Source: CAD feature listing. Evaluate the final solid. Frame: model axes, mm. A direction names the side the tool comes from. Round coordinates to 2 decimals unless told otherwise and drop trailing zeros. Loops run counter-clockwise (first coordinate to the right, second up) from the corner with the lowest first, then second, coordinate; pieces in that order, holes last. Notation, with made-up numbers: (-6.75, 1.25) - (3.25, 1.25) arc R27 ccw to (3.25, 37.25) - close; hole circle Ø11 at (-14.5, -28.5). An arc over 180 degrees is marked (long way). One line per question, with ' | ' between items.
from build123d import *

# Parameters (mm, degrees)
EXTRUDE_1_DEPTH     = 20
CUT_EXTRUDE_1_REACH = 71.771
SKETCH_2_R          = 1.55
SKETCH_2_R_2        = 11.5
CUT_EXTRUDE_2_REACH = 71.771
SKETCH_3_R          = 1.55
FILLET_1_R          = 5


with BuildPart() as part:
    # 草图1 → 凸台-拉伸1 (new, symmetric)
    with BuildSketch(Plane(origin=(0, 0, 0), x_dir=(0, 0, -1), z_dir=(1, 0, 0))):
        Polygon((0, 0), (0, 52), (3, 52), (3, 3), (42, 3), (42, 0), align=None)
    extrude(amount=EXTRUDE_1_DEPTH, both=True)

    # 草图2 → 切除-拉伸1 (cut, up to next)
    with BuildSketch(Plane.XY, mode=Mode.PRIVATE) as cut_extrude_1_sk1:
        with Locations((15.5, 46.5)):
            Circle(SKETCH_2_R)
    cut_extrude_1_tool1 = extrude(cut_extrude_1_sk1.sketch, amount=-CUT_EXTRUDE_1_REACH, mode=Mode.PRIVATE) & part.part
    # 草图2 → 切除-拉伸1 (cut, up to next)
    with BuildSketch(Plane.XY, mode=Mode.PRIVATE) as cut_extrude_1_sk2:
        with Locations((15.5, 15.5)):
            Circle(SKETCH_2_R)
    cut_extrude_1_tool2 = extrude(cut_extrude_1_sk2.sketch, amount=-CUT_EXTRUDE_1_REACH, mode=Mode.PRIVATE) & part.part
    # 草图2 → 切除-拉伸1 (cut, up to next)
    with BuildSketch(Plane.XY, mode=Mode.PRIVATE) as cut_extrude_1_sk3:
        with Locations(Location((-15.5, 15.5, 0), (0, 0, 90))):
            Circle(SKETCH_2_R)
    cut_extrude_1_tool3 = extrude(cut_extrude_1_sk3.sketch, amount=-CUT_EXTRUDE_1_REACH, mode=Mode.PRIVATE) & part.part
    # 草图2 → 切除-拉伸1 (cut, up to next)
    with BuildSketch(Plane.XY, mode=Mode.PRIVATE) as cut_extrude_1_sk4:
        with Locations(Location((-15.5, 46.5, 0), (0, 0, 90))):
            Circle(SKETCH_2_R)
    cut_extrude_1_tool4 = extrude(cut_extrude_1_sk4.sketch, amount=-CUT_EXTRUDE_1_REACH, mode=Mode.PRIVATE) & part.part
    # 草图2 → 切除-拉伸1 (cut, up to next)
    with BuildSketch(Plane.XY, mode=Mode.PRIVATE) as cut_extrude_1_sk5:
        with Locations((0, 31)):
            Circle(SKETCH_2_R_2)
    cut_extrude_1_tool5 = extrude(cut_extrude_1_sk5.sketch, amount=-CUT_EXTRUDE_1_REACH, mode=Mode.PRIVATE) & part.part
    add(cut_extrude_1_tool1.solids().sort_by_distance((15.5, 46.5, 0))[0], mode=Mode.SUBTRACT)
    add(cut_extrude_1_tool2.solids().sort_by_distance((15.5, 15.5, 0))[0], mode=Mode.SUBTRACT)
    add(cut_extrude_1_tool3.solids().sort_by_distance((-15.5, 15.5, 0))[0], mode=Mode.SUBTRACT)
    add(cut_extrude_1_tool4.solids().sort_by_distance((-15.5, 46.5, 0))[0], mode=Mode.SUBTRACT)
    add(cut_extrude_1_tool5.solids().sort_by_distance((0, 31, 0))[0], mode=Mode.SUBTRACT)

    # 草图3 → 切除-拉伸2 (cut, up to next)
    with BuildSketch(Plane(origin=(0, 0, 0), x_dir=(1, 0, 0), z_dir=(0, 1, 0)), mode=Mode.PRIVATE) as cut_extrude_2_sk1:
        with Locations(Location((15, 33, 0), (0, 0, 270))):
            Circle(SKETCH_3_R)
    cut_extrude_2_tool1 = extrude(cut_extrude_2_sk1.sketch, amount=CUT_EXTRUDE_2_REACH, mode=Mode.PRIVATE) & part.part
    # 草图3 → 切除-拉伸2 (cut, up to next)
    with BuildSketch(Plane(origin=(0, 0, 0), x_dir=(1, 0, 0), z_dir=(0, 1, 0)), mode=Mode.PRIVATE) as cut_extrude_2_sk2:
        with Locations(Location((15, 9, 0), (0, 0, 270))):
            Circle(SKETCH_3_R)
    cut_extrude_2_tool2 = extrude(cut_extrude_2_sk2.sketch, amount=CUT_EXTRUDE_2_REACH, mode=Mode.PRIVATE) & part.part
    # 草图3 → 切除-拉伸2 (cut, up to next)
    with BuildSketch(Plane(origin=(0, 0, 0), x_dir=(1, 0, 0), z_dir=(0, 1, 0)), mode=Mode.PRIVATE) as cut_extrude_2_sk3:
        with Locations(Location((-15, 9, 0), (0, 0, 90))):
            Circle(SKETCH_3_R)
    cut_extrude_2_tool3 = extrude(cut_extrude_2_sk3.sketch, amount=CUT_EXTRUDE_2_REACH, mode=Mode.PRIVATE) & part.part
    # 草图3 → 切除-拉伸2 (cut, up to next)
    with BuildSketch(Plane(origin=(0, 0, 0), x_dir=(1, 0, 0), z_dir=(0, 1, 0)), mode=Mode.PRIVATE) as cut_extrude_2_sk4:
        with Locations(Location((-15, 33, 0), (0, 0, 90))):
            Circle(SKETCH_3_R)
    cut_extrude_2_tool4 = extrude(cut_extrude_2_sk4.sketch, amount=CUT_EXTRUDE_2_REACH, mode=Mode.PRIVATE) & part.part
    add(cut_extrude_2_tool1.solids().sort_by_distance((15, 0, -33))[0], mode=Mode.SUBTRACT)
    add(cut_extrude_2_tool2.solids().sort_by_distance((15, 0, -9))[0], mode=Mode.SUBTRACT)
    add(cut_extrude_2_tool3.solids().sort_by_distance((-15, 0, -9))[0], mode=Mode.SUBTRACT)
    add(cut_extrude_2_tool4.solids().sort_by_distance((-15, 0, -33))[0], mode=Mode.SUBTRACT)

    # 圆角1
    fillet_1_edges = [part.edges().sort_by_distance(p)[0] for p in [
        (-20, 52, -1.5),
        (20, 52, -1.5),
        (20, 1.5, -42),
        (-20, 1.5, -42),
    ]]
    fillet(fillet_1_edges, radius=FILLET_1_R)


solid = part.part
1. Contact query for flat-ended pins moving along their axis: P1, Ø1, axis at x = 4, z = -30, coming from the -Y side; P2, Ø19.5, axis at x = -3, z = -27.5, coming from the +Y side; P3, Ø1, axis at x = 13, y = 18, coming from the -Z side. Output: stop coordinate, or through.
Worked out:
P1: stops at y = 0 | P2: stops at y = 3 | P3: stops at z = -3
2. Access query for faces 5 (the flat face through (-9, 22, -3)), 6 (the flat face through (-4, 20, 0)). Directions: +Z, -Z, +X, -X, +Y, -Y. A direction counts if a zero-diameter tool reaches every point of the face in a straight line with its end or side. Return the directions, or none.
Worked out:
face 5: -Z, +X, -X, +Y | face 6: +Z, +X, -X, +Y, -Y
3. Mould query, pull axis Y, two halves, no side actions, for faces 1 (the flat face through (0, 3, -22)), 2 (the cylindrical face through (-15.466, 1.479, -34.478)), 3 (the cylindrical face through (14.36, 16.55, -1.48)), 4 (the cylindrical face through (15.164, 44.987, -1.479)). Classes: released by +Y, released by -Y, zero draft, split by the parting line, or undercut.
Worked out:
face 1: released by +Y | face 2: zero draft | face 3: undercut | face 4: undercut
4. Section query A-A, the plane x = 0. Return loops of the section in (y, z), plus the area to 3 significant figures.
Worked out:
outline: (0, -42) - (3, -42) - (3, -3) - (19.5, -3) - (19.5, 0) - (0, 0) - close; (42.5, -3) - (52, -3) - (52, 0) - (42.5, 0) - close | area: 204 mm2
5. Material intervals for probe 1 along X at (y, z) = (0.7, -9); probe 2 along Z at (x, y) = (-15, 1); probe 3 along Y at (x, z) = (-15, -1), sorted ascending.
Worked out:
probe 1: x = -20 to -16.55, -13.45 to 13.45, 16.55 to 20 | probe 2: z = -42 to -34.55, -31.45 to -10.55, -7.45 to 0 | probe 3: y = 0 to 14.03, 16.97 to 45.03, 47.97 to 52
6. Section query D-D, the plane x = -4. Return loops of the section in (y, z), plus the area to 3 significant figures.
Worked out:
outline: (0, -42) - (3, -42) - (3, -3) - (20.22, -3) - (20.22, 0) - (0, 0) - close; (41.78, -3) - (52, -3) - (52, 0) - (41.78, 0) - close | area: 208 mm2
7. Section query C-C, the plane y = 27. Return loops of the section in (x, z), plus the area to 3 significant figures.
Worked out:
outline: (-20, -3) - (-10.78, -3) - (-10.78, 0) - (-20, 0) - close; (10.78, -3) - (20, -3) - (20, 0) - (10.78, 0) - close | area: 55.3 mm2
8. Section query B-B, the plane z = -33. Return loops of the section in (x, y).
Worked out:
outline: (-20, 0) - (-16.55, 0) - (-16.55, 3) - (-20, 3) - close; (-13.45, 0) - (13.45, 0) - (13.45, 3) - (-13.45, 3) - close; (16.55, 0) - (20, 0) - (20, 3) - (16.55, 3) - close
